Check sheet for the modelled part. Datum: model origin and axes. Units: mm. Coordinates: 2 decimals unless noted, no trailing zeros. Loops run counter-clockwise (first coordinate to the right, second up) from the corner with the lowest first, then second, coordinate; pieces in that order, holes last.
```python
from build123d import *

# Parameters (mm, degrees)
SKETCH1_W           = 12
SKETCH1_H           = 87.5
SKETCH1_R           = 1.5
BOSS_EXTRUDE1_DEPTH = 5


with BuildPart() as part:
    # Sketch1 → Boss-Extrude1 (new, symmetric)
    with BuildSketch(Plane(origin=(0, 0, 0), x_dir=(0, 0, -1), z_dir=(1, 0, 0))):
        with Locations((0, 40)):
            Rectangle(SKETCH1_W, SKETCH1_H)
        with Locations((0, 80)):
            Circle(SKETCH1_R, mode=Mode.SUBTRACT)
        Circle(SKETCH1_R, mode=Mode.SUBTRACT)
    extrude(amount=BOSS_EXTRUDE1_DEPTH, both=True)


solid = part.part
```
1) Section check B-B on y = 0. Enter the section's corners in (x, z).
Answer sheet:
outline: (-5, -6) - (5, -6) - (5, -1.5) - (-5, -1.5) - close; (-5, 1.5) - (5, 1.5) - (5, 6) - (-5, 6) - close
2) Section check A-A on z = 0. Enter the section's corners in (x, y).
Answer sheet:
outline: (-5, -3.75) - (5, -3.75) - (5, -1.5) - (-5, -1.5) - close; (-5, 1.5) - (5, 1.5) - (5, 78.5) - (-5, 78.5) - close; (-5, 81.5) - (5, 81.5) - (5, 83.75) - (-5, 83.75) - close
3) Mould release check, pull along Y, two halves, no side actions. Record for faces 1 (the flat face through (0, -3.75, 0)), 2 (the cylindrical face through (-0.07, 0.07, 1.5)), 3 (the cylindrical face through (-0.07, 81.265, -0.806)), 4 (the flat face through (0, 39, 6)): +Y half, -Y half, draft (parallel to the pull), parting line (faces both ways), or undercut.
Answer sheet:
face 1: -Y half
face 2: undercut
face 3: undercut
face 4: draft
4) Scan lines: line 1 (Y direction, x = -1.25, z = 0); line 2 (Y direction, x = 2.5, z = 0.5); line 3 (Z direction, x = 2.75, y = 80). Record each from-to range of solid material in increasing order.
Answer sheet:
line 1: y = -3.75 to -1.5, 1.5 to 78.5, 81.5 to 83.75
line 2: y = -3.75 to -1.41, 1.41 to 78.59, 81.41 to 83.75
line 3: z = -6 to -1.5, 1.5 to 6
